The listing builds one solid part. Answer for the finished solid, in the listing's coordinates (mm). A direction names the side the tool comes from. Give positions to 0.01 mm unless a question says otherwise; leave off trailing zeros. Write each loop counter-clockwise with the first axis right and the second up, starting at its lowest first coordinate (ties: lowest second). Pieces come first, ordered by that corner, then holes. Notation, with made-up numbers: M 84,72 L 96,72 A27 cw 96,101 Z; hole C -25,85 d6. An arc over 180 degrees is marked long. Return JSON: item names as keys, results as strings.
Autodesk Inventor part; units mm, degrees
ref_plane "YZ Plane" through (0, 0, 0) normal (1, 0, 0) x (0, 1, 0)
ref_plane "XZ Plane" through (0, 0, 0) normal (0, 1, 0) x (-1, 0, 0)
ref_plane "XY Plane" through (0, 0, 0) normal (0, 0, 1) x (1, 0, 0)
sketch "Sketch1" plane through (0, 0, 0) normal (0, 0, 1) x (1, 0, 0)
  line L0 (-81, 75) -> (81, 75)
  line L1 (81, 75) -> (81, -75)
  line L2 (81, -75) -> (-81, -75)
  line L3 (-81, -75) -> (-81, 75)
  point P0 (0, 0)
  point P1 (-81, 0)
  point P2 (0, 75)
  dimension "d0" = 162
  dimension "d1" = 150
extrude "Extrusion1" add sketch "Sketch1" along normal blind 4
sketch "Sketch3" plane through (81, -75, 0) normal (1, 0, 0) x (0, 0, -1)
  line L0 (-4, 0) -> (-4, 150)
  line L1 (-4, 105.918) -> (0, 105.918)
  line L2 (0, 105.918) -> (0, 55.918)
  line L3 (0, 55.918) -> (-4, 55.918)
  line L4 (-4, 55.918) -> (-4, 105.918)
  point P0 (0, 75)
  dimension "d7" = 50
extrude "Extrusion3" add sketch "Sketch3" along normal blind 4
mirror "Mirror2" about plane through (0, 0, 0) normal (1, 0, 0) of "Extrusion3"
properties part number "Rampa"
Item 1: Given pin 1 Ø1.2 at (x, z) = (-84, 2) entering from +Y; pin 2 Ø1.2 at (x, z) = (83, 2.5) entering from -Y; pin 3 Ø1.5 at (y, z) = (59, 1) entering from -X, each flat-ended and moving along its own axis, determine where each tip first touches the part or whether it passes through.
Geometry results:
{"pin 1": "stops at y = 30.92", "pin 2": "stops at y = -19.08", "pin 3": "stops at x = -81"}
Item 2: A cutting plane is placed at B-B, the plane y = 58.5. Write down the section's boundary in (x, z), plus the area to 3 significant figures.
Geometry results:
{"outline": "M -81,0 L 81,0 L 81,4 L -81,4 Z", "area": "648 mm2"}
Item 3: Find the intervals of material crossed by line 1 (X direction, y = 63.5, z = 1.2), in increasing order.
Geometry results:
{"line 1": "x = -81 to 81"}
Item 4: Which of the six approach directions +Z, -Z, +X, -X, +Y, -Y give full straight-line access (tool end or side, diameter ignored) to faces 1 (the flat face through (-81, -47, 2)), 2 (the flat face through (81, 53, 2)), 3 (the flat face through (-83, 30.918, 2)), 4 (the flat face through (81, -47, 2)), 5 (the flat face through (85, 6, 2))?
Geometry results:
{"face 1": "+Z, -Z, -X, -Y", "face 2": "+Z, -Z, +X, +Y", "face 3": "+Z, -Z, -X, +Y", "face 4": "+Z, -Z, +X, -Y", "face 5": "+Z, -Z, +X, +Y, -Y"}
Item 5: A cutting plane is placed at A-A, the plane z = 3.3. Write down the section's boundary in (x, y).
Geometry results:
{"outline": "M -85,-19.08 L -81,-19.08 L -81,-75 L 81,-75 L 81,-19.08 L 85,-19.08 L 85,30.92 L 81,30.92 L 81,75 L -81,75 L -81,30.92 L -85,30.92 Z"}
